Answer from the drawing. Dimensions are ordinates in mm from the lowest x, y and z of the part. Coordinates: 2 decimals unless noted, no trailing zeros. Write each loop counter-clockwise with the first axis right and the second up, starting at its lowest first coordinate (ties: lowest second). Pieces come first, ordered by that corner, then holes. Notation, with made-up numbers: (39.5, 50) - (75.5, 50) arc R24 ccw to (75.5, 65) - close; hole circle Ø6 at (23, 23). An arc over 180 degrees is marked (long way). Use a Markdown table: item, result.
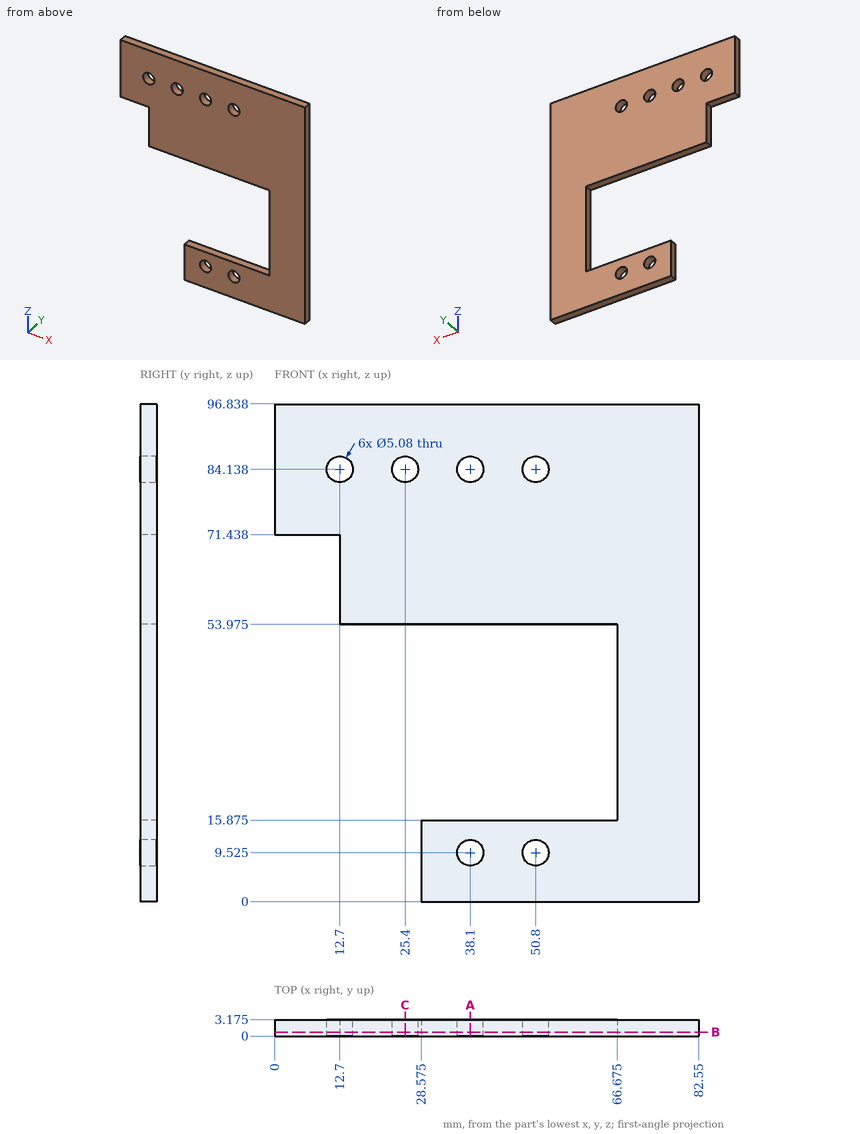
(1) Each of these flat-tipped pins is pushed along its axis until it touches: P1, Ø6.5, axis at x = 50.8, z = 9.525, coming from the +Y side (1 decimal); P2, Ø4, axis at x = 50.8, z = 84.14, coming from the -Y side; P3, Ø1, axis at x = 5, y = 1, coming from the -Z side; P4, Ø1, axis at x = 18.5, y = 1.5, coming from the -Z side (1 decimal). Where does it stop, or does it pass through?
Report:
| item | result |
|---|---|
| P1 | stops at y = 3.2 |
| P2 | passes through |
| P3 | stops at z = 71.44 |
| P4 | stops at z = 54 |
(2) A cutting plane is placed at C-C, the plane x = 25.4. Write down the section's boundary in (y, z) (1 decimal).
Report:
| item | result |
|---|---|
| outline | (0, 54) - (3.2, 54) - (3.2, 81.6) - (0, 81.6) - close; (0, 86.7) - (3.2, 86.7) - (3.2, 96.8) - (0, 96.8) - close |
(3) A cutting plane is placed at A-A, the plane x = 38.1. Write down the section's boundary in (y, z) (1 decimal), and give its area (3 significant figures).
Report:
| item | result |
|---|---|
| outline | (0, 0) - (3.2, 0) - (3.2, 7) - (0, 7) - close; (0, 12.1) - (3.2, 12.1) - (3.2, 15.9) - (0, 15.9) - close; (0, 54) - (3.2, 54) - (3.2, 81.6) - (0, 81.6) - close; (0, 86.7) - (3.2, 86.7) - (3.2, 96.8) - (0, 96.8) - close |
| area | 154 mm² |
(4) Straight lines are drawn through the part: L1, parallel to Z at x = 55, y = 0.6 (1 decimal); L2, parallel to Z at x = 19.5, y = 3.05 (1 decimal); L3, parallel to X at y = 2.35, z = 59. For each, find the intervals that lie inside material, in ascending order.
Report:
| item | result |
|---|---|
| L1 | z = 0 to 15.9, 54 to 96.8 |
| L2 | z = 54 to 96.8 |
| L3 | x = 12.7 to 82.55 |
(5) A cutting plane is placed at B-B, the plane y = 0.75. Count the separate pieces of the cut face and the enclosed holes in it, and give its area (3 significant figures).
Report:
| item | result |
|---|---|
| separate pieces | 1 |
| enclosed holes | 6 |
| area | 4,660 mm² |
